Verification items for the finished model (mm, model axes). A direction names the side the tool comes from. Coordinates: 2 decimals unless noted, no trailing zeros. Write each loop counter-clockwise with the first axis right and the second up, starting at its lowest first coordinate (ties: lowest second). Pieces come first, ordered by that corner, then holes. Notation, with made-up numbers: M 2.5,39.25 L 59.5,39.25 A14 cw 59.5,56.25 Z; hole C -5.5,51 d1. An arc over 180 degrees is marked long. One line per item, written item: value.
Autodesk Inventor part; units mm, degrees
ref_plane "YZ Plane" through (0, 0, 0) normal (1, 0, 0) x (0, 1, 0)
ref_plane "XZ Plane" through (0, 0, 0) normal (0, 1, 0) x (-1, 0, 0)
ref_plane "XY Plane" through (0, 0, 0) normal (0, 0, 1) x (1, 0, 0)
sketch "Sketch1" plane through (0, 0, 0) normal (0, 0, 1) x (1, 0, 0)
  line L0 (12.7, 0) -> (165.1, 0)
  line L1 (177.8, 12.7) -> (177.8, 88.9)
  line L2 (165.1, 101.6) -> (12.7, 101.6)
  line L3 (0, 88.9) -> (0, 12.7)
  arc A0 (12.7, 101.6) -> (0, 88.9) centre (12.7, 88.9) ccw
  arc A1 (0, 12.7) -> (12.7, 0) centre (12.7, 12.7) ccw
  arc A2 (165.1, 0) -> (177.8, 12.7) centre (165.1, 12.7) ccw
  arc A3 (177.8, 88.9) -> (165.1, 101.6) centre (165.1, 88.9) ccw
  circle A4 centre (12.7, 88.9) radius 5.08
  circle A5 centre (165.1, 88.9) radius 5.08
  circle A6 centre (165.1, 12.7) radius 5.08
  circle A7 centre (12.7, 12.7) radius 5.08
  circle A8 centre (63.5, 88.9) radius 5.08
  circle A9 centre (114.3, 88.9) radius 5.08
  circle A10 centre (63.5, 12.7) radius 5.08
  circle A11 centre (114.3, 12.7) radius 5.08
  arc A12 (111.125, 32.8395) -> (111.125, 68.7605) centre (133.35, 50.8) ccw
  arc A13 (66.675, 68.7605) -> (66.675, 32.8395) centre (44.45, 50.8) ccw
  arc A14 (66.675, 32.8395) -> (111.125, 32.8395) centre (88.9, 50.8) ccw
  arc A15 (111.125, 68.7605) -> (66.675, 68.7605) centre (88.9, 50.8) ccw
  point P0 (0, 0)
  point P1 (177.8, 0)
  point P2 (0, 101.6)
  dimension "d0" = 101.6
  dimension "d1" = 177.8
  dimension "d2" = 12.7
  dimension "d3" = 10.16
  dimension "d4" = 10.16
  dimension "d15" = 50.8
  dimension "d17" = 50.8
  dimension "d18" = 88.9
  dimension "d19" = 57.15
  dimension "d20" = 44.45
  dimension "d21" = 57.15
  dimension "d22" = 44.45
extrude "Extrusion1" add sketch "Sketch1" along normal blind 6.35
properties part number "HW 8 Part 5"
Item 1: Scan lines: line 1 (Y direction, x = 165.1, z = 3.75); line 2 (Y direction, x = 114.3, z = 4); line 3 (X direction, y = 50.8, z = 2) (3 decimals). Record each from-to range of solid material in increasing order.
The answers:
line 1: y = 0 to 7.62, 17.78 to 83.82, 93.98 to 101.6
line 2: y = 0 to 7.62, 17.78 to 29.5, 72.1 to 83.82, 93.98 to 101.6
line 3: x = 0 to 15.875, 161.925 to 177.8
Item 2: Draft check along Y on faces 3 (the face through (15.89, 49.82, 3.13)), 4 (the face through (177.8, 50, 3)), 5 (the face through (3.62, 97.78, 3.13)). Enter one of: released by +Y, released by -Y, zero draft, split by the parting line, or undercut.
The answers:
face 3: undercut
face 4: zero draft
face 5: released by +Y
Item 3: Cross-section at B-B, the plane y = 50.8. Enter the section's corners in (x, z) (3 decimals), and give its area (3 significant figures).
The answers:
outline: M 0,0 L 15.875,0 L 15.875,6.35 L 0,6.35 Z; M 161.925,0 L 177.8,0 L 177.8,6.35 L 161.925,6.35 Z
area: 202 mm²
Item 4: Cross-section at D-D, the plane x = 114.3. Enter the section's corners in (y, z).
The answers:
outline: M 0,0 L 7.62,0 L 7.62,6.35 L 0,6.35 Z; M 17.78,0 L 29.5,0 L 29.5,6.35 L 17.78,6.35 Z; M 72.1,0 L 83.82,0 L 83.82,6.35 L 72.1,6.35 Z; M 93.98,0 L 101.6,0 L 101.6,6.35 L 93.98,6.35 Z
Item 5: Cross-section at C-C, the plane z = 3. Give the number of separate pieces and of enclosed holes in the cut face, and give its area (3 significant figures).
The answers:
separate pieces: 1
enclosed holes: 9
area: 10,200 mm²
Item 6: Cross-section at A-A, the plane x = 133.35. Enter the section's corners in (y, z) (3 decimals), and give its area (3 significant figures).
The answers:
outline: M 0,0 L 22.225,0 L 22.225,6.35 L 0,6.35 Z; M 79.375,0 L 101.6,0 L 101.6,6.35 L 79.375,6.35 Z
area: 282 mm²
Item 7: Go/stop test with a flat-tipped pin: P1, Ø13, axis at x = 63.5, y = 12.7, coming from the -Z side. Record where the tip stops, or that it passes through.
The answers:
P1: stops at z = 0
Item 8: Access from +Z, -Z, +X, -X, +Y, -Y to the whole of each face (thin tool, end or side, straight path). Record for faces 1 (the face through (90, 101.6, 3)), 2 (the face through (88.544, 79.373, 3.131)).
The answers:
face 1: +Z, -Z, +X, -X, +Y
face 2: +Z, -Z
